Read the model definition and answer for the solid it produces. Units are mm, in the model's axes. A direction names the side the tool comes from. Coordinates: 2 decimals unless noted, no trailing zeros. Order: outer loops, then holes, each group sorted by start corner. A loop starts at its lowest first (then second) coordinate and runs counter-clockwise, first axis right, second up. Notation, with made-up numbers: (-2, 79) - (37, 79) arc R21 cw to (37, 102) - close; hole circle Ø9 at (21, -0.75). An arc over 180 degrees is marked (long way). Write item = value, one per line.
from build123d import *

# Parameters (mm, degrees)
SKETCH1_W               = 96.89
SKETCH1_H               = 90.17
PCB_DEPTH               = 1.57
SKETCH2_R               = 2
M3_MOUNTING_HOLES_DEPTH = 1.57
SKETCH5_W               = 0.5
SKETCH5_H               = 90.17
CUT_EXTRUDE1_DEPTH      = 2.57
SKETCH8_R               = 1.25
RPI_MOUNTING_HOLE_DEPTH = 10
SKETCH9_R               = 2
POWERADAPTERHOLES_DEPTH = 10
SKETCH10_W              = 5
SKETCH10_H              = 2
DSUB_HOLDER_DEPTH       = 10
FILLET2_R               = 2
DSUB_FIELDS_REACH       = 69.17
SKETCH11_R              = 1.5


with BuildPart() as part:
    # Sketch1 → PCB (new body)
    with BuildSketch(Plane(origin=(0, 0, 0), x_dir=(1, 0, 0), z_dir=(0, 1, 0))):
        with Locations((16.200949951, 63.633996534)):
            Rectangle(SKETCH1_W, SKETCH1_H)
    extrude(amount=PCB_DEPTH)

    # Sketch2 → M3 Mounting Holes (cut)
    with BuildSketch(Plane(origin=(0, 1.57, 0), x_dir=(1, 0, 0), z_dir=(0, 1, 0))):
        with Locations((59.565949951, 24.898996534)):
            Circle(SKETCH2_R)
        with Locations((-26.164050049, 27.438996534)):
            Circle(SKETCH2_R)
        with Locations((-26.164050049, 101.098996534)):
            Circle(SKETCH2_R)
        with Locations((59.565949951, 103.638996534)):
            Circle(SKETCH2_R)
    extrude(amount=-M3_MOUNTING_HOLES_DEPTH, mode=Mode.SUBTRACT)

    # Sketch5 → Cut-Extrude1 (cut, through all)
    with BuildSketch(Plane(origin=(0, 1.57, 0), x_dir=(1, 0, 0), z_dir=(0, 1, 0))):
        with Locations((-31.994050049, 63.633996534)):
            Rectangle(SKETCH5_W, SKETCH5_H)
        with Locations((64.395949951, 63.633996534)):
            Rectangle(SKETCH5_W, SKETCH5_H)
    extrude(amount=-CUT_EXTRUDE1_DEPTH, mode=Mode.SUBTRACT)

    # Sketch8 → RPi mounting hole (cut)
    with BuildSketch(Plane(origin=(0, 1.57, 0), x_dir=(1, 0, 0), z_dir=(0, 1, 0))):
        with Locations((3.255949951, 45.718996534)):
            Circle(SKETCH8_R)
        with Locations((52.255949951, 45.718996534)):
            Circle(SKETCH8_R)
        with Locations((4.255949951, 103.718996534)):
            Circle(SKETCH8_R)
        with Locations((53.255949951, 103.718996534)):
            Circle(SKETCH8_R)
    extrude(amount=-RPI_MOUNTING_HOLE_DEPTH, mode=Mode.SUBTRACT)

    # Sketch9 → PowerAdapterHoles (cut)
    with BuildSketch(Plane(origin=(0, 1.57, 0), x_dir=(1, 0, 0), z_dir=(0, 1, 0))):
        with Locations((-18.744050049, 91.548996534)):
            Circle(SKETCH9_R)
        with Locations((-18.744050049, 53.548996534)):
            Circle(SKETCH9_R)
    extrude(amount=-POWERADAPTERHOLES_DEPTH, mode=Mode.SUBTRACT)

    # Sketch10 → DSub Holder (add)
    with BuildSketch(Plane(origin=(0, 1.57, 0), x_dir=(1, 0, 0), z_dir=(0, 1, 0))):
        with Locations((-28.244050049, 42.548996534)):
            Rectangle(SKETCH10_W, SKETCH10_H)
        with Locations((-3.244050049, 42.548996534)):
            Rectangle(SKETCH10_W, SKETCH10_H)
    extrude(amount=DSUB_HOLDER_DEPTH)

    # Fillet2
    fillet2_edges = [part.edges().sort_by_distance(p)[0] for p in [
        (-3.244050049, 1.57, -43.548996534),
        (-28.244050049, 1.57, -43.548996534),
    ]]
    fillet(fillet2_edges, radius=FILLET2_R)

    # Sketch11 → DSub Fields (cut, up to next)
    with BuildSketch(Plane.XY.offset(-41.548996534), mode=Mode.PRIVATE) as dsub_fields_sk1:
        with Locations((-28.244050049, 8.57)):
            Circle(SKETCH11_R)
    dsub_fields_tool1 = extrude(dsub_fields_sk1.sketch, amount=-DSUB_FIELDS_REACH, mode=Mode.PRIVATE) & part.part
    add(dsub_fields_tool1.solids().sort_by_distance((-28.24405, 8.57, -41.548997))[0], mode=Mode.SUBTRACT)
    # Sketch11 → DSub Fields (cut, up to next)
    with BuildSketch(Plane.XY.offset(-41.548996534), mode=Mode.PRIVATE) as dsub_fields_sk2:
        with Locations((-3.254050049, 8.57)):
            Circle(SKETCH11_R)
    dsub_fields_tool2 = extrude(dsub_fields_sk2.sketch, amount=-DSUB_FIELDS_REACH, mode=Mode.PRIVATE) & part.part
    add(dsub_fields_tool2.solids().sort_by_distance((-3.25405, 8.57, -41.548997))[0], mode=Mode.SUBTRACT)


solid = part.part
1) The part is cut by section A-A (y = 5.5). Determine the outline of the cut face in (x, z).
Returned:
outline = (-30.74, -43.55) - (-25.74, -43.55) - (-25.74, -41.55) - (-30.74, -41.55) - close; (-5.74, -43.55) - (-0.74, -43.55) - (-0.74, -41.55) - (-5.74, -41.55) - close
2) Straight lines are drawn through the part: line 1 along X through (y, z) = (2.25, -43); line 2 along Y through (x, z) = (7, -93.5). For each, find the intervals that lie inside material, in ascending order. Write a range as from..to.
Returned:
line_1 = -30.74..-25.74, -5.74..-0.74
line_2 = 0..1.57
3) The part is cut by section C-C (x = 43.5). Determine the outline of the cut face in (y, z), and give its area (3 significant figures).
Returned:
outline = (0, -108.72) - (1.57, -108.72) - (1.57, -18.55) - (0, -18.55) - close
area = 142 mm^2
4) For faces 1 (the face through (-28, 6, -41.549)), 2 (the face through (16, 0, -64)), 3 (the face through (-30.744, 6, -43)), 4 (the face through (-5.744, 6, -43)), 5 (the face through (-28.3, 6.6, -43.549)), determine the directions among +Z, -Z, +X, -X, +Y, -Y from which every point of the face is accessible in a straight line to the end or side of a thin tool.
Returned:
face_1 = +Z, +X, -X, +Y
face_2 = +Z, -Z, +X, -X, -Y
face_3 = +Z, -Z, -X, +Y
face_4 = +Z, -Z, +Y
face_5 = -Z, +X, -X, +Y
5) The part is cut by section B-B (z = -85.5). Determine the outline of the cut face in (x, y).
Returned:
outline = (-31.74, 0) - (64.15, 0) - (64.15, 1.57) - (-31.74, 1.57) - close
6) Determine the mould class of faces 6 (the face through (-3, 6, -41.549)), 7 (the face through (-26.598, 0.796, -99.147)), 8 (the face through (-25.744, 6, -43)), 9 (the face through (-3.21, 2.14, -44.15)) for opening direction Z: pulls with the +Z half, pulls with the -Z half, needs draft (parallel to the pull), parting line crosses it, or undercut.
Returned:
face_6 = pulls with the +Z half
face_7 = undercut
face_8 = needs draft
face_9 = pulls with the -Z half
7) Flat-ended cylindrical pins translate along their axes: pin 1 Ø5 at (x, z) = (59.57, -103.64) entering from +Y; pin 2 Ø3 at (x, z) = (52.26, -45.72) entering from -Y; pin 3 Ø3 at (y, z) = (4.5, -43.5) entering from +X; pin 4 Ø2.5 at (x, y) = (-2, 8.5) entering from -Z. Find the tip coordinate at first contact, or state that the pin passes through.
Returned:
pin_1 = 1.57
pin_2 = 0
pin_3 = -0.74
pin_4 = -43.55
